```python
from build123d import *

# Parameters (mm, degrees)
F0_W     = 60
F0_H     = 45
F1_DEPTH = 2
F3_D     = 3


with BuildPart() as f1:
    # F0 (on Top) → F1 (new body)
    with BuildSketch(Plane.XY):
        Rectangle(F0_W, F0_H)
    extrude(amount=-F1_DEPTH)

    # F3 (through all)
    with Locations(Plane.XY):
        with Locations((-23, 12.5), (23, 12.5), (0, -15.5)):
            Hole(F3_D / 2)


solid = f1.part
```
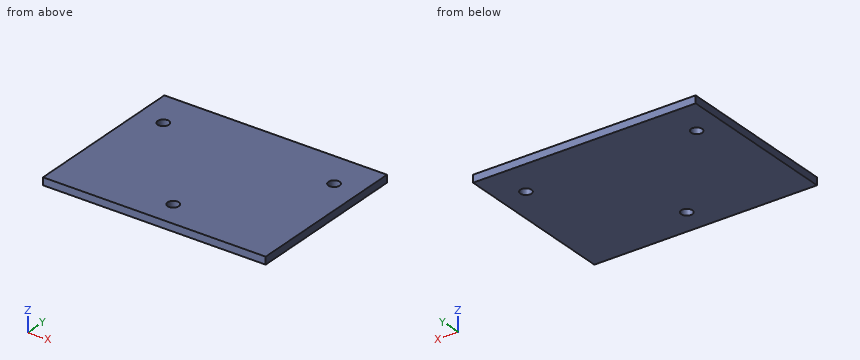
Build history of the part. All positions in model axes, mm. Coordinates: 2 decimals unless noted, no trailing zeros. Write each loop counter-clockwise with the first axis right and the second up, starting at its lowest first coordinate (ties: lowest second). Pieces come first, ordered by that corner, then holes.
1. Band-saw the part on C-C, the plane x = -23. Give the cut face in (y, z).
Answer block:
outline: (-22.5, -2) - (11, -2) - (11, 0) - (-22.5, 0) - close; (14, -2) - (22.5, -2) - (22.5, 0) - (14, 0) - close
2. Drill centre lines: probe 1 along Y at (x, z) = (0, -1.2); probe 2 along Y at (x, z) = (-23, -0.55); probe 3 along X at (y, z) = (13.5, -1.4). Where is each one in solid material? Low to high.
Answer block:
probe 1: y = -22.5 to -17, -14 to 22.5
probe 2: y = -22.5 to 11, 14 to 22.5
probe 3: x = -30 to -24.12, -21.88 to 21.88, 24.12 to 30
3. Band-saw the part on A-A, the plane y = 12.5. Give the cut face in (x, z), and give its area (3 significant figures).
Answer block:
outline: (-30, -2) - (-24.5, -2) - (-24.5, 0) - (-30, 0) - close; (-21.5, -2) - (21.5, -2) - (21.5, 0) - (-21.5, 0) - close; (24.5, -2) - (30, -2) - (30, 0) - (24.5, 0) - close
area: 108 mm2
4. Band-saw the part on B-B, the plane y = -15.5. Give the cut face in (x, z), and give its area (3 significant figures).
Answer block:
outline: (-30, -2) - (-1.5, -2) - (-1.5, 0) - (-30, 0) - close; (1.5, -2) - (30, -2) - (30, 0) - (1.5, 0) - close
area: 114 mm2
